from build123d import *

# Parameters (mm, degrees)
SKETCH_1_R                = 30
EXTRUDE_1_DEPTH           = 75
EXTRUDE_1_DEPTH_BACK      = 50
SKETCH_10_W               = 30
SKETCH_10_H               = 30
CUT_EXTRUDE_8_DEPTH       = 45.1
SKETCH_10_2_W             = 30
SKETCH_10_2_H             = 30
CUT_EXTRUDE_9_DEPTH       = 10
CUT_EXTRUDE_9_DEPTH_BACK  = 113
CUT_EXTRUDE_10_DEPTH      = 54
SKETCH_12_R               = 28
CUT_EXTRUDE_11_DEPTH      = 72
CUT_EXTRUDE_11_DEPTH_BACK = 55
SKETCH_13_W               = 13
SKETCH_13_H               = 23.5
CUT_EXTRUDE_12_DEPTH      = 54
SKETCH_14_W               = 5
SKETCH_14_H               = 5
EXTRUDE_2_DEPTH           = 1
EXTRUDE_2_DEPTH_BACK      = 4
SKETCH_15_R               = 1.1
CUT_EXTRUDE_13_DEPTH      = 4
CUT_EXTRUDE_13_DEPTH_BACK = 5


with BuildPart() as part:
    # Sketch 1 → Extrude 1 (new body, two sides)
    with BuildSketch(Plane(origin=(0, 0, 0), x_dir=(1, 0, 0), z_dir=(0, 1, 0))) as extrude_1_sk:
        Circle(SKETCH_1_R)
    extrude(amount=EXTRUDE_1_DEPTH)
    extrude(extrude_1_sk.sketch, amount=-EXTRUDE_1_DEPTH_BACK)

    # Sketch 10 → Cut-Extrude 8 (cut)
    with BuildSketch(Plane(origin=(0, 75, 0), x_dir=(1, 0, 0), z_dir=(0, 1, 0))):
        Rectangle(SKETCH_10_W, SKETCH_10_H)
    extrude(amount=-CUT_EXTRUDE_8_DEPTH, mode=Mode.SUBTRACT)

    # Sketch 10_2 → Cut-Extrude 9 (cut, two sides)
    with BuildSketch(Plane(origin=(0, 75, 0), x_dir=(1, 0, 0), z_dir=(0, 1, 0))) as cut_extrude_9_sk:
        Rectangle(SKETCH_10_2_W, SKETCH_10_2_H)
    extrude(amount=CUT_EXTRUDE_9_DEPTH, mode=Mode.SUBTRACT)
    extrude(cut_extrude_9_sk.sketch, amount=-CUT_EXTRUDE_9_DEPTH_BACK, mode=Mode.SUBTRACT)

    # Sketch 11 → Cut-Extrude 10 (cut)
    with BuildSketch(Plane(origin=(0, 0, 0), x_dir=(1, 0, 0), z_dir=(0, 1, 0))):
        with BuildLine():
            Line((25.732316415, 15.422317981), (-26.32585788, 14.385729278))
            ThreePointArc((-26.32585788, 14.385729278), (0.597245261, -29.994054379), (25.732316415, 15.422317981))
        make_face()
    extrude(amount=-CUT_EXTRUDE_10_DEPTH, mode=Mode.SUBTRACT)

    # Sketch 12 → Cut-Extrude 11 (cut, two sides)
    with BuildSketch(Plane(origin=(0, 0, 0), x_dir=(1, 0, 0), z_dir=(0, 1, 0))) as cut_extrude_11_sk:
        Circle(SKETCH_12_R)
    extrude(amount=CUT_EXTRUDE_11_DEPTH, mode=Mode.SUBTRACT)
    extrude(cut_extrude_11_sk.sketch, amount=-CUT_EXTRUDE_11_DEPTH_BACK, mode=Mode.SUBTRACT)

    # Sketch 13 → Cut-Extrude 12 (cut)
    with BuildSketch(Plane.XY):
        with Locations((0, -24.25)):
            Rectangle(SKETCH_13_W, SKETCH_13_H)
    extrude(amount=-CUT_EXTRUDE_12_DEPTH, mode=Mode.SUBTRACT)

    # Sketch 14 → Extrude 2 (add, two sides)
    with BuildSketch(Plane.XY.offset(-28)) as extrude_2_sk:
        with Locations((0, -38.5)):
            Rectangle(SKETCH_14_W, SKETCH_14_H)
        with Locations((0, -10)):
            Rectangle(SKETCH_14_W, SKETCH_14_H)
    extrude(amount=EXTRUDE_2_DEPTH)
    extrude(extrude_2_sk.sketch, amount=-EXTRUDE_2_DEPTH_BACK)

    # Sketch 15 → Cut-Extrude 13 (cut, two sides)
    with BuildSketch(Plane.XY.offset(-28)) as cut_extrude_13_sk:
        with Locations((0, -10)):
            Circle(SKETCH_15_R)
        with Locations((0, -38.5)):
            Circle(SKETCH_15_R)
    extrude(amount=CUT_EXTRUDE_13_DEPTH, mode=Mode.SUBTRACT)
    extrude(cut_extrude_13_sk.sketch, amount=-CUT_EXTRUDE_13_DEPTH_BACK, mode=Mode.SUBTRACT)


solid = part.part
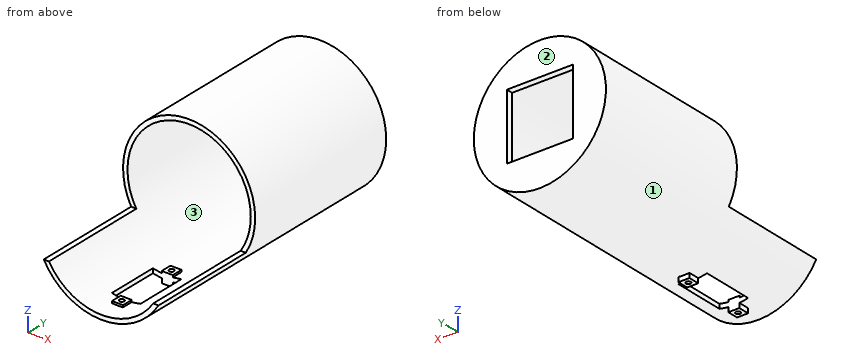
CAD build for the part. Positions are in the model's coordinates, mm. Face numbers are marked on the shaded views. Coordinates: 2 decimals unless noted, no trailing zeros. Order: outer loops, then holes, each group sorted by start corner. A loop starts at its lowest first (then second) coordinate and runs counter-clockwise, first axis right, second up.
Item 1: Pin check, flat tips, straight feed: pin 1 Ø0.7 at (y, z) = (-11, -27.5) entering from -X; pin 2 Ø1.1 at (y, z) = (-39, -31) entering from +X; pin 3 Ø12 at (y, z) = (15.5, 8.5) entering from -X. Stop position of each tip, or through.
Check sheet entries:
pin 1: stops at x = -12.76
pin 2: stops at x = 2.5
pin 3: stops at x = -29.9
Item 2: Band-saw the part on C-C on x = 20.5. List the corners of the cut face in (y, z).
Check sheet entries:
outline: (-50, -21.9) - (75, -21.9) - (75, 21.9) - (0, 21.9) - (0, 19.07) - (72, 19.07) - (72, -19.07) - (-50, -19.07) - close
Item 3: Band-saw the part on A-A on z = 0. List the corners of the cut face in (x, y).
Check sheet entries:
outline: (-30, 0) - (-28, 0) - (-28, 72) - (-15, 72) - (-15, 75) - (-30, 75) - close; (15, 72) - (28, 72) - (28, 0) - (30, 0) - (30, 75) - (15, 75) - close
Item 4: Two-plate mould, pull along Z, no slides. Class the marked faces 1, 2 and 3: +Z half, -Z half, draft (parallel to the pull), parting line (faces both ways), or undercut.
Check sheet entries:
face 1: parting line
face 2: draft
face 3: undercut
Item 5: Drill centre lines: L1, parallel to Y at x = 0, z = -29; L2, parallel to X at y = -10, z = -30.5; L3, parallel to Z at x = 0, y = 24. Where is each one in solid material? Low to high.
Check sheet entries:
L1: y = -50 to -39.6, -37.4 to -36, -12.5 to -11.1, -8.9 to 75
L2: x = -2.5 to -1.1, 1.1 to 2.5
L3: z = -30 to -28, 28 to 30
Item 6: Band-saw the part on B-B on x = -4. List the corners of the cut face in (y, z).
Check sheet entries:
outline: (-50, -29.73) - (-36, -29.73) - (-36, -27.71) - (-50, -27.71) - close; (-12.5, -29.73) - (75, -29.73) - (75, -15) - (72, -15) - (72, -27.71) - (-12.5, -27.71) - close; (0, 27.71) - (72, 27.71) - (72, 15) - (75, 15) - (75, 29.73) - (0, 29.73) - close
Item 7: Band-saw the part on D-D on z = -8. List the corners of the cut face in (x, y).
Check sheet entries:
outline: (-28.91, 0) - (-26.83, 0) - (-26.83, 72) - (-15, 72) - (-15, 75) - (-28.91, 75) - close; (15, 72) - (26.83, 72) - (26.83, 0) - (28.91, 0) - (28.91, 75) - (15, 75) - close
